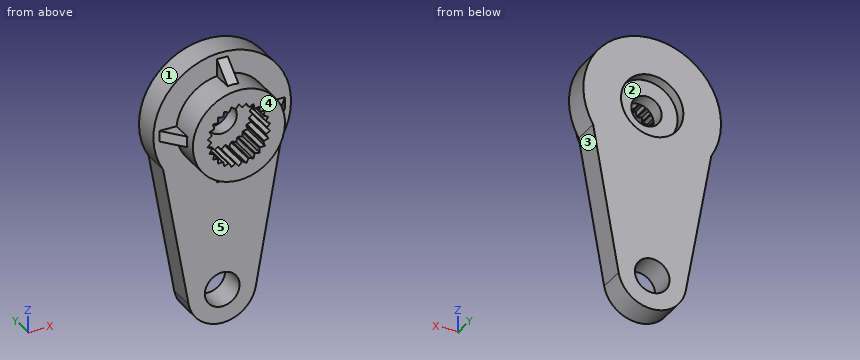
```python
from build123d import *

# Parameters (mm, degrees)
BASES_R             = 6.35
BASE_DEPTH          = 5.4
TOPBORES_R          = 1.4
TOP_BORE_DEPTH      = 11.478788098
HORN_START          = -2.5
HORN_HALF_DEPTH     = 2.5
HORNATTACHS_R       = 1.6
HORN_ATTACH_DEPTH   = 21.913031822
TOOTH_DEPTH         = 3
TOOTH_CP_COUNT      = 26
BOTTOMBORES_R       = 2.6
BOTTOM_BORE_DEPTH   = 3
HOLDINGSHAFTS_R     = 6.35
HOLDINGSHAFTS_R_2   = 4.25
HOLDING_SHAFT_DEPTH = 2.9
RIB_DEPTH           = 0.5
RIB_CP_COUNT        = 4
SKETCH1_R           = 2.875
CUT_EXTRUDE1_DEPTH  = 1


with BuildPart() as part:
    # BaseS → BASE (new body)
    with BuildSketch(Plane(origin=(0, 0, 0), x_dir=(1, 0, 0), z_dir=(0, 1, 0))):
        with Locations(Location((0, 0, 0), (0, 0, 90))):
            Circle(BASES_R)
    extrude(amount=BASE_DEPTH)

    # TopBoreS → TOP BORE (cut, through all)
    with BuildSketch(Plane(origin=(0, 5.4, 0), x_dir=(1, 0, 0), z_dir=(0, 1, 0))):
        with Locations(Location((0, 0, 0), (0, 0, 270))):
            Circle(TOPBORES_R)
    extrude(amount=-TOP_BORE_DEPTH, mode=Mode.SUBTRACT)

    # HornHalfS → HORN HALF (add)
    with BuildSketch(Plane(origin=(0, 5.4, 0), x_dir=(1, 0, 0), z_dir=(0, 1, 0)).offset(HORN_START)):
        with BuildLine():
            Line((-3.102144422, 16.57699176), (-5.450702003, 3.257659846))
            ThreePointArc((-5.450702003, 3.257659846), (0, 6.35), (5.450702003, 3.257659846))
            Line((5.450702003, 3.257659846), (3.102144422, 16.57699176))
            ThreePointArc((3.102144422, 16.57699176), (0, 19.18), (-3.102144422, 16.57699176))
        make_face()
    extrude(amount=HORN_HALF_DEPTH)

    # HornAttachS → HORN ATTACH (cut, through all)
    with BuildSketch(Plane(origin=(0, 5.4, 0), x_dir=(1, 0, 0), z_dir=(0, 1, 0))):
        with Locations(Location((0, 16.03, 0), (0, 0, 270))):
            Circle(HORNATTACHS_R)
    extrude(amount=-HORN_ATTACH_DEPTH, mode=Mode.SUBTRACT)

    # ToothS → TOOTH (cut)
    with BuildSketch(Plane.XZ):
        with BuildLine():
            Line((0, -2.9), (0.262912611, -2.586672952))
            ThreePointArc((0.262912611, -2.586672952), (0, -2.6), (-0.262912611, -2.586672952))
            Line((-0.262912611, -2.586672952), (0, -2.9))
        make_face()
    tooth = extrude(amount=-TOOTH_DEPTH, mode=Mode.SUBTRACT)

    # TOOTH CP: TOOTH ×26 about axis
    tooth_cp_axis = Axis((0, 0, 0), (0, 1, 0))
    for i in range(1, TOOTH_CP_COUNT):
        add(tooth.rotate(tooth_cp_axis, i * 360 / TOOTH_CP_COUNT), mode=Mode.SUBTRACT)

    # BottomBoreS → BOTTOM BORE (cut)
    with BuildSketch(Plane(origin=(0, 0, 0), x_dir=(-1, 0, 0), z_dir=(0, -1, 0))):
        Circle(BOTTOMBORES_R)
    extrude(amount=-BOTTOM_BORE_DEPTH, mode=Mode.SUBTRACT)

    # HoldingShaftS → HOLDING SHAFT (cut)
    with BuildSketch(Plane.XZ):
        Circle(HOLDINGSHAFTS_R)
        with Locations(Location((0, 0, 0), (0, 0, 270))):
            Circle(HOLDINGSHAFTS_R_2, mode=Mode.SUBTRACT)
    extrude(amount=-HOLDING_SHAFT_DEPTH, mode=Mode.SUBTRACT)

    # RibS → RIB (add, symmetric)
    with BuildSketch(Plane.XY):
        Polygon((4.21, 1), (5.804289299, 2.9), (4.21, 2.9), (4.16, 2.9), (4.16, 1), align=None)
    rib = extrude(amount=RIB_DEPTH, both=True)

    # RIB CP: RIB ×4 about axis
    rib_cp_axis = Axis((0, 0, 0), (0, 1, 0))
    for i in range(1, RIB_CP_COUNT):
        add(rib.rotate(rib_cp_axis, i * 360 / RIB_CP_COUNT))

    # Sketch1 → Cut-Extrude1 (cut)
    with BuildSketch(Plane(origin=(0, 5.4, 0), x_dir=(1, 0, 0), z_dir=(0, 1, 0))):
        with Locations(Location((0, 0, 0), (0, 0, 270))):
            Circle(SKETCH1_R)
    extrude(amount=-CUT_EXTRUDE1_DEPTH, mode=Mode.SUBTRACT)


solid = part.part
```
Could you check a few things on this model? Use its own coordinates, in mm. Face numbers are marked on the shaded views. A direction names the side the tool comes from. Give positions to 0.01 mm unless a question says otherwise; leave off trailing zeros. Loops run counter-clockwise (first coordinate to the right, second up) from the corner with the lowest first, then second, coordinate; pieces in that order, holes last. Notation, with made-up numbers: (0, 13.25) - (25, 13.25) arc R32 cw to (25, 48.25) - close; hole circle Ø10 at (3.5, -39.5). An arc over 180 degrees is marked (long way). Use one line per item in the form item = value.
1. Thinking about a two-plate mould opening in X: for the marked faces 1, 2 and 3, which applies, released by +X, released by -X, zero draft, split by the parting line, or undercut?
Response values:
face_1 = split by the parting line
face_2 = undercut
face_3 = released by +X
2. On a 3-axis mill with a long thin cutter (end or side, diameter ignored), from which of +Z, -Z, +X, -X, +Y, -Y can I reach the whole of each face in a straight line? I mean the marked faces 4 and 5. Say none if no direction works.
Response values:
face_4 = +Z, -Z, +X, -X, -Y
face_5 = -Y
3. I want a section at C-C (z = 3.75). Please give me the cut outline in (x, y).
Response values:
outline = (-5.12, 2.9) - (-2, 2.9) - (-2, 0) - (2, 0) - (2, 2.9) - (5.12, 2.9) - (5.12, 5.4) - (-5.12, 5.4) - close
4. I want a section at A-A (z = -16.03). Please give me the cut outline in (x, y).
Response values:
outline = (-3.2, 2.9) - (-1.6, 2.9) - (-1.6, 5.4) - (-3.2, 5.4) - close; (1.6, 2.9) - (3.2, 2.9) - (3.2, 5.4) - (1.6, 5.4) - close
5. I need wall thicknesses on probe 1 along X at (y, z) = (5.15, 0) (3 decimals); probe 2 along Z at (x, y) = (-2.75, 2.85); probe 3 along Z at (x, y) = (-0.75, 5.1). Which ranges of each line are inside material? Lowest first, please.
Response values:
probe_1 = -6.35 to -2.875, 2.875 to 6.35
probe_2 = -3.24 to -0.43, -0.21 to 0.21, 0.43 to 3.24
probe_3 = -19.09 to -17.44, -14.62 to -2.78, 2.78 to 6.31
6. I want a section at B-B (x = -3.75). Please give me the cut outline in (y, z).
Response values:
outline = (0, -2) - (2.9, -2) - (2.9, -12.9) - (5.4, -12.9) - (5.4, 5.12) - (2.9, 5.12) - (2.9, 2) - (0, 2) - close
7. I'm going to push flat-ended pins straight in: pin 1 Ø1.5 at (x, z) = (3.5, -11.5) entering from -Y; pin 2 Ø3.5 at (x, z) = (0, 0) entering from -Y; pin 3 Ø1.7 at (x, y) = (5.5, 2) entering from +Z. Where does each tip first touch, or does it pass through?
Response values:
pin_1 = 2.9
pin_2 = 3
pin_3 = 0.5
